Geometry check sheet. Reference: the model listing, model coordinates, mm. A direction names the side the tool comes from. Round coordinates to 2 decimals unless told otherwise and drop trailing zeros. Order: outer loops, then holes, each group sorted by start corner. A loop starts at its lowest first (then second) coordinate and runs counter-clockwise, first axis right, second up. Notation, with made-up numbers: (4.25, 70) - (21.25, 70) arc R17 cw to (21.25, 99) - close; hole circle Ø5 at (36, 58). An arc over 180 degrees is marked (long way). Use a Markdown table: item, result. Add a question column.
(1) Section check D-D on y = 9. Record the boundary of the cut face in (x, z).
(2) Thickness scan on line 1 along Z through (x, y) = (8, 0); line 2 along X through (y, z) = (3.45, 0); line 3 along Y through (x, z) = (10, -1.75). Record the ranges inside material, lowest first. Write a range as [from, to].
(3) Section check B-B on y = 0. Record the boundary of the cut face in (x, z), then the cut area to 3 significant figures.
(4) Section check C-C on x = 9.5. Give the number of separate pieces and of enclosed holes in the cut face, then the cut area to 3 significant figures.
(5) Access from +Z, -Z, +X, -X, +Y, -Y to the whole of each face (thin tool, end or side, straight path). Record for faces 1 (the face through (7.4, -1.89, 11.24)), 2 (the face through (7.395, -7.171, -7.145)), 3 (the face through (7.4, -11.27, 1.91)).
(6) Gauge pin test, flat ends, axial feed: P1, Ø0.9, axis at y = 7, z = -1, coming from the -X side; P2, Ø4, axis at x = 12, y = 2.5, coming from the +Z side; P3, Ø4.5, axis at x = 5.5, z = 0, coming from the -Y side. Record the tip position at first contact, or that the pin passes through.
(7) Mould release check, pull along Y, two halves, no side actions. Record for faces 4 (the face through (7.4, -6.62, 9.32)), 5 (the face through (7.4, -3.7, -13.12)), 6 (the face through (7.4, -3.1, 0.1)), 7 (the face through (7.395, 6.666, 11.865)): released by +Y, released by -Y, zero draft, split by the parting line, or undercut.
(8) Section check A-A on z = 0. Record the boundary of the cut face in (x, y), then the cut area to 3 significant figures.
```python
from build123d import *

# Parameters (mm, degrees)
F0_R     = 3.1
F0_W     = 3.1
F0_H     = 7.2
F1_DEPTH = 15
F2_DEPTH = 11
F3_R     = 2.05
F4_DEPTH = 5
F5_DEPTH = 25


with BuildPart() as f1:
    # F0 (on Right) → F1 (new body)
    with BuildSketch(Plane.YZ):
        with BuildLine():
            ThreePointArc((2.704842, 12.353416), (1.898315, 11.252912), (1.266883, 10.043413))
            ThreePointArc((1.266883, 10.043413), (0, 10.123), (-1.266883, 10.043413))
            ThreePointArc((-1.266883, 10.043413), (-1.898315, 11.252912), (-2.704842, 12.353416))
            ThreePointArc((-2.704842, 12.353416), (-3.690651, 13.113822), (-4.718141, 13.816887))
            Line((-4.718141, 13.816887), (-6.433785, 13.106244))
            ThreePointArc((-6.433785, 13.106244), (-6.663188, 11.882557), (-6.822573, 10.647796))
            ThreePointArc((-6.822573, 10.647796), (-6.614699, 9.299322), (-6.205943, 7.997587))
            ThreePointArc((-6.205943, 7.997587), (-7.158042, 7.158042), (-7.997587, 6.205943))
            ThreePointArc((-7.997587, 6.205943), (-9.299322, 6.614699), (-10.647796, 6.822573))
            ThreePointArc((-10.647796, 6.822573), (-11.882557, 6.663188), (-13.106244, 6.433785))
            Line((-13.106244, 6.433785), (-13.816887, 4.718141))
            ThreePointArc((-13.816887, 4.718141), (-13.113822, 3.690651), (-12.353416, 2.704842))
            ThreePointArc((-12.353416, 2.704842), (-11.252912, 1.898315), (-10.043413, 1.266883))
            ThreePointArc((-10.043413, 1.266883), (-10.123, 0), (-10.043413, -1.266883))
            ThreePointArc((-10.043413, -1.266883), (-11.252912, -1.898315), (-12.353416, -2.704842))
            ThreePointArc((-12.353416, -2.704842), (-13.113822, -3.690651), (-13.816887, -4.718141))
            Line((-13.816887, -4.718141), (-13.106244, -6.433785))
            ThreePointArc((-13.106244, -6.433785), (-11.882557, -6.663188), (-10.647796, -6.822573))
            ThreePointArc((-10.647796, -6.822573), (-9.299322, -6.614699), (-7.997587, -6.205943))
            ThreePointArc((-7.997587, -6.205943), (-7.158042, -7.158042), (-6.205943, -7.997587))
            ThreePointArc((-6.205943, -7.997587), (-6.614699, -9.299322), (-6.822573, -10.647796))
            ThreePointArc((-6.822573, -10.647796), (-6.663188, -11.882557), (-6.433785, -13.106244))
            Line((-6.433785, -13.106244), (-4.718141, -13.816887))
            ThreePointArc((-4.718141, -13.816887), (-3.690651, -13.113822), (-2.704842, -12.353416))
            ThreePointArc((-2.704842, -12.353416), (-1.898315, -11.252912), (-1.266883, -10.043413))
            ThreePointArc((-1.266883, -10.043413), (0, -10.123), (1.266883, -10.043413))
            ThreePointArc((1.266883, -10.043413), (1.898315, -11.252912), (2.704842, -12.353416))
            ThreePointArc((2.704842, -12.353416), (3.690651, -13.113822), (4.718141, -13.816887))
            Line((4.718141, -13.816887), (6.433785, -13.106244))
            ThreePointArc((6.433785, -13.106244), (6.663188, -11.882557), (6.822573, -10.647796))
            ThreePointArc((6.822573, -10.647796), (6.614699, -9.299322), (6.205943, -7.997587))
            ThreePointArc((6.205943, -7.997587), (7.158042, -7.158042), (7.997587, -6.205943))
            ThreePointArc((7.997587, -6.205943), (9.299322, -6.614699), (10.647796, -6.822573))
            ThreePointArc((10.647796, -6.822573), (11.882557, -6.663188), (13.106244, -6.433785))
            Line((13.106244, -6.433785), (13.816887, -4.718141))
            ThreePointArc((13.816887, -4.718141), (13.113822, -3.690651), (12.353416, -2.704842))
            ThreePointArc((12.353416, -2.704842), (11.252912, -1.898315), (10.043413, -1.266883))
            ThreePointArc((10.043413, -1.266883), (10.123, 0), (10.043413, 1.266883))
            ThreePointArc((10.043413, 1.266883), (11.252912, 1.898315), (12.353416, 2.704842))
            ThreePointArc((12.353416, 2.704842), (13.113822, 3.690651), (13.816887, 4.718141))
            Line((13.816887, 4.718141), (13.106244, 6.433785))
            ThreePointArc((13.106244, 6.433785), (11.882557, 6.663188), (10.647796, 6.822573))
            ThreePointArc((10.647796, 6.822573), (9.299322, 6.614699), (7.997587, 6.205943))
            ThreePointArc((7.997587, 6.205943), (7.158042, 7.158042), (6.205943, 7.997587))
            ThreePointArc((6.205943, 7.997587), (6.614699, 9.299322), (6.822573, 10.647796))
            ThreePointArc((6.822573, 10.647796), (6.663188, 11.882557), (6.433785, 13.106244))
            Line((6.433785, 13.106244), (4.718141, 13.816887))
            ThreePointArc((4.718141, 13.816887), (3.690651, 13.113822), (2.704842, 12.353416))
        make_face()
        Circle(F0_R, mode=Mode.SUBTRACT)
        with Locations((6.55, 0)):
            Rectangle(F0_W, F0_H, mode=Mode.SUBTRACT)
        with Locations((6.55, 0)):
            Rectangle(F0_W, F0_H)
    extrude(amount=F1_DEPTH)

    # F0 (on Right) → F2 (cut)
    with BuildSketch(Plane.YZ):
        with Locations((6.55, 0)):
            Rectangle(F0_W, F0_H)
    extrude(amount=F2_DEPTH, mode=Mode.SUBTRACT)

    # F3 (on face) → F4 (cut)
    with BuildSketch(Plane(origin=(0, 5, 0), x_dir=(-1, 0, 0), z_dir=(0, 1, 0))):
        with Locations((-5.5, 0)):
            Circle(F3_R)
    extrude(amount=-F4_DEPTH, mode=Mode.SUBTRACT)

    # F3 (on face) → F5 (cut)
    with BuildSketch(Plane(origin=(0, 5, 0), x_dir=(-1, 0, 0), z_dir=(0, 1, 0))):
        with Locations((-5.5, 0)):
            Circle(F3_R)
    extrude(amount=F5_DEPTH, mode=Mode.SUBTRACT)


solid = f1.part
```
Check sheet entries:
| question | item | result |
|---|---|---|
| 1 | outline | (0, -6.54) - (15, -6.54) - (15, 6.54) - (0, 6.54) - close; hole circle Ø4.1 at (5.5, 0) |
| 2 | line 1 | z = [-10.12, -3.1], [3.1, 10.12] |
| 2 | line 2 | x = [0, 3.45], [7.55, 15] |
| 2 | line 3 | y = [-11.01, -2.56], [2.56, 5], [8.1, 11.01] |
| 3 | outline | (0, -10.12) - (15, -10.12) - (15, -3.1) - (0, -3.1) - close; (0, 3.1) - (15, 3.1) - (15, 10.12) - (0, 10.12) - close |
| 3 | area | 211 mm2 |
| 4 | separate pieces | 1 |
| 4 | enclosed holes | 2 |
| 4 | area | 422 mm2 |
| 5 | face 1 | +Z, +X, -X |
| 5 | face 2 | +X, -X |
| 5 | face 3 | +X, -X, -Y |
| 6 | P1 | stops at x = 11 |
| 6 | P2 | stops at z = 13.67 |
| 6 | P3 | stops at y = -11.78 |
| 7 | face 4 | released by -Y |
| 7 | face 5 | undercut |
| 7 | face 6 | undercut |
| 7 | face 7 | released by +Y |
| 8 | outline | (0, -10.12) - (15, -10.12) - (15, -3.1) - (0, -3.1) - close; (0, 3.1) - (3.45, 3.1) - (3.45, 5) - (0, 5) - close; (0, 8.1) - (3.45, 8.1) - (3.45, 10.12) - (0, 10.12) - close; (7.55, 3.1) - (15, 3.1) - (15, 10.12) - (7.55, 10.12) - (7.55, 8.1) - (11, 8.1) - (11, 5) - (7.55, 5) - close |
| 8 | area | 161 mm2 |
